Autodesk Inventor part; units mm, degrees
ref_plane "YZ Plane" through (0, 0, 0) normal (1, 0, 0) x (0, 1, 0)
ref_plane "XZ Plane" through (0, 0, 0) normal (0, 1, 0) x (-1, 0, 0)
ref_plane "XY Plane" through (0, 0, 0) normal (0, 0, 1) x (1, 0, 0)
sketch "Sketch1" plane through (0, 0, 0) normal (1, 0, 0) x (0, 1, 0)
  line L0 (7, 51) -> (0, 51)
  line L1 (0, 41) -> (0, -41)
  line L2 (0, -51) -> (7, -51)
  line L3 (7, 51) -> (-3, 51)
  line L4 (-3, 51) -> (-3, 41)
  line L5 (-3, 41) -> (0, 41)
  line L6 (7, 41) -> (7, 51)
  line L7 (7, 51) -> (7, 51)
  line L8 (10, 48) -> (10, 46)
  line L9 (10, 46) -> (7, 46)
  line L10 (7, 46) -> (7, 51)
  line L11 (7, 8) -> (10, 8)
  line L12 (10, 8) -> (10, -8)
  line L13 (10, -8) -> (7, -8)
  line L14 (-3, -41) -> (0, -41)
  line L15 (10, -46) -> (7, -46)
  line L16 (7, -51) -> (-3, -51)
  line L17 (-3, -51) -> (-3, -41)
  line L18 (7, -51) -> (0, -51)
  line L19 (7, -41) -> (7, -46)
  line L20 (7, -51) -> (7, -51)
  line L21 (10, -48) -> (10, -46)
  line L22 (7, -46) -> (7, -8)
  line L23 (7, 8) -> (7, 51)
  arc A0 (10, 48) -> (7, 51) centre (7, 48) ccw
  arc A1 (7, -51) -> (10, -48) centre (7, -48) ccw
  point P0 (0, 0)
  point P1 (10, -51)
  point P2 (0, 51)
  dimension "d10" = 10
  dimension "d11" = 10
  dimension "d13" = 5
  dimension "d15" = 43
  dimension "d16" = 59
  dimension "d17" = 102
  dimension "d18" = 13
  dimension "d19" = 3
  dimension "d20" = 3
extrude "Extrusion1" add sketch "Sketch1" along normal blind 82
sketch "Sketch2" plane through (0, 0, 0) normal (0, 1, 0) x (-1, 0, 0)
  line L0 (0, 51) -> (0, 48)
  line L1 (0, 51) -> (0, 17)
  line L2 (0, 41) -> (0, -41)
  line L3 (0, 17) -> (-22, 17)
  circle A0 centre (-22, 17) radius 3
  line L4 (0, -41) -> (0, -51)
  line L5 (0, -51) -> (0, -17)
  line L6 (0, -17) -> (-22, -17)
  line L7 (0, -41) -> (-82, -41)
  line L8 (0, -51) -> (-82, -51)
  line L9 (-82, -51) -> (-82, -17)
  line L10 (-82, 41) -> (-82, -41)
  line L11 (-82, -17) -> (-60, -17)
  line L12 (-82, 51) -> (-82, 48)
  line L13 (-82, 51) -> (-82, 17)
  line L14 (-82, 8) -> (-82, 46)
  line L15 (-82, 17) -> (-60, 17)
  circle A1 centre (-22, -17) radius 3
  circle A2 centre (-60, -17) radius 3
  circle A3 centre (-60, 17) radius 3
  point P0 (0, 0)
  dimension "d23" = 34
  dimension "d24" = 22
  dimension "d25" = 6
  dimension "d26" = 34
  dimension "d27" = 22
  dimension "d28" = 34
  dimension "d29" = 22
  dimension "d30" = 34
  dimension "d31" = 22
  dimension "d32" = 6
  dimension "d33" = 6
  dimension "d34" = 6
extrude "Extrusion2" cut sketch "Sketch2" along normal mid plane 62 contours A3 | A2 | A1 | A0
properties material "Polycarbonate, Clear"
Design review of the part built by this model. Coordinates are the model's own, in mm. A direction names the side the tool comes from. Coordinates: 2 decimals unless noted, no trailing zeros. Order: outer loops, then holes, each group sorted by start corner. A loop starts at its lowest first (then second) coordinate and runs counter-clockwise, first axis right, second up.
1) Take a section at B-B, the plane x = 60. Give the boundary of the cut face in (y, z), and give its area (3 significant figures).
2) Clearance check with flat-ended pins moving along their axes: pin 1 (0.9 mm diameter, centred on x = 28, y = 8.5, fed in from -Z); pin 2 (5 mm diameter, centred on x = 20.5, z = 14, fed in from -Y); pin 3 (11.5 mm diameter, centred on x = 58, z = -33.5, fed in from +Y). State where each tip first meets the part, or that it passes through.
3) Take a section at C-C, the plane y = 8.75. Give the boundary of the cut face in (x, z), and give its area (3 significant figures).
4) For faces 1 (the flat face through (40, 9, -8)), 2 (the flat face through (0, 3, 1)), 3 (the flat face through (40, 0, 1)), list the 3-axis set-ups (+Z, -Z, +X, -X, +Y, -Y) from which the entire face can be reached by the end or side of a thin tool; tool diameter is ignored.
5) Take a section at D-D, the plane x = 47. Give the boundary of the cut face in (y, z), and give its area (3 significant figures).
6) Mouldability with a two-part tool opening along Z and no side actions: class faces 4 (the flat face through (82, 3, 1)), 5 (the cylindrical face through (63, 4, -17)), 6 (the cylindrical face through (40.43, 9.14, -50.1)) as +Z half, -Z half, draft (parallel to the pull), parting line (faces both ways), or undercut.
7) Wall thickness on line 1 along Z through (x, y) = (60, 5); line 2 along Z through (x, y) = (63.5, -2.25); line 3 along Z through (x, y) = (62, 8): over which ranges is each line inside the solid? List them lowest first.
8) Take a section at A-A, the plane z = 17. Give the boundary of the cut face in (x, y), and give its area (3 significant figures).
Returned:
1. outline: (-3, -51) - (7, -51) arc R3 ccw to (10, -48) - (10, -46) - (7, -46) - (7, -20) - (0, -20) - (0, -41) - (-3, -41) - close; (-3, 41) - (0, 41) - (0, 20) - (7, 20) - (7, 46) - (10, 46) - (10, 48) arc R3 ccw to (7, 51) - (-3, 51) - close; (0, -14) - (7, -14) - (7, -8) - (10, -8) - (10, 8) - (7, 8) - (7, 14) - (0, 14) - close
1. area: 764 mm2
2. pin 1: stops at z = -50.81
2. pin 2: stops at y = 0
2. pin 3: stops at y = 7
3. outline: (0, -50.44) - (82, -50.44) - (82, -46) - (0, -46) - close; (0, -8) - (82, -8) - (82, 8) - (0, 8) - close; (0, 46) - (82, 46) - (82, 50.44) - (0, 50.44) - close
3. area: 2,040 mm2
4. face 1: +X, -X, +Y
4. face 2: +Z, -Z, -X, +Y, -Y
4. face 3: +X, -X, -Y
5. outline: (-3, -51) - (7, -51) arc R3 ccw to (10, -48) - (10, -46) - (7, -46) - (7, -8) - (10, -8) - (10, 8) - (7, 8) - (7, 46) - (10, 46) - (10, 48) arc R3 ccw to (7, 51) - (-3, 51) - (-3, 41) - (0, 41) - (0, -41) - (-3, -41) - close
5. area: 848 mm2
6. face 4: draft
6. face 5: undercut
6. face 6: -Z half
7. line 1: z = -51 to -20, -14 to 14, 20 to 51
7. line 2: z = -51 to -41, 41 to 51
7. line 3: z = -50.83 to -46, -8 to 8, 46 to 50.83
8. outline: (0, 0) - (19, 0) - (19, 7) - (0, 7) - close; (25, 0) - (57, 0) - (57, 7) - (25, 7) - close; (63, 0) - (82, 0) - (82, 7) - (63, 7) - close
8. area: 490 mm2
